Build history of the part. All positions in model axes, mm. Round coordinates to 2 decimals unless told otherwise and drop trailing zeros. Loops run counter-clockwise (first coordinate to the right, second up) from the corner with the lowest first, then second, coordinate; pieces in that order, holes last. Notation, with made-up numbers: (69, 54) - (110, 54) arc R22 cw to (110, 90) - close; hole circle Ø3 at (53, 68). An arc over 180 degrees is marked (long way). Put each result on its own line as item: value. Start each with the question number.
from build123d import *

# Parameters (mm, degrees)
F0_W     = 15
F0_H     = 5.08
F1_DEPTH = 5.08
F2_DEPTH = 25
F4_DEPTH = 50
F5_W     = 15
F5_H     = 5.08
F6_DEPTH = 5.08


# Not quite as in the source:
# - a feature names something its author has since deleted; it is built from what else it names


with BuildPart() as f1:
    # F0 (on Front) → F1 (new body)
    with BuildSketch(Plane.XZ):
        Polygon((-75.7, 0), (0, 0), (0, 50), (-104.7, 50), (-133.1023774395, 50), (-184.7, 50), (-184.7, 101.5976225605), (-184.7, 130), (-234.7, 130), (-234.7, 0), (-219.7, 0), (-210.7, 0), (-195.7, 0), (-186.7, 0), (-171.7, 0), (-162.7, 0), (-147.7, 0), (-138.7, 0), (-123.7, 0), (-114.7, 0), (-99.7, 0), (-90.7, 0), align=None)
        with Locations((-83.2, -2.54)):
            Rectangle(F0_W, F0_H)
        Polygon((-133.1023774395, 50), (-104.7, 50), (-184.7, 130), (-184.7, 101.5976225605), align=None)
        with Locations((-107.2, -2.54)):
            Rectangle(F0_W, F0_H)
        with Locations((-131.2, -2.54)):
            Rectangle(F0_W, F0_H)
        with Locations((-227.2, -2.54)):
            Rectangle(F0_W, F0_H)
        with Locations((-155.2, -2.54)):
            Rectangle(F0_W, F0_H)
        with Locations((-203.2, -2.54)):
            Rectangle(F0_W, F0_H)
        with Locations((-179.2, -2.54)):
            Rectangle(F0_W, F0_H)
    extrude(amount=F1_DEPTH)

    # F2 (add): a face of the model
    f2_faces = [f1.faces().sort_by_distance(p)[0] for p in [
        (-209.7, -2.54, 130),
    ]]
    extrude(f2_faces, amount=F2_DEPTH)

    # F3 (on face) → F4 (cut)
    with BuildSketch(Plane(origin=(0, 0, 0), x_dir=(1, 0, 0), z_dir=(0, 0, -1))):
        Polygon((0, 0), (0, 5.08), (-2.9329393675, 0), align=None)
    extrude(amount=-F4_DEPTH, mode=Mode.SUBTRACT)

    # F5 (on face) → F6 (join)
    with BuildSketch(Plane.XY.offset(50)):
        with Locations((-82.2, -2.54)):
            Rectangle(F5_W, F5_H)
    extrude(amount=F6_DEPTH)


solid = f1.part
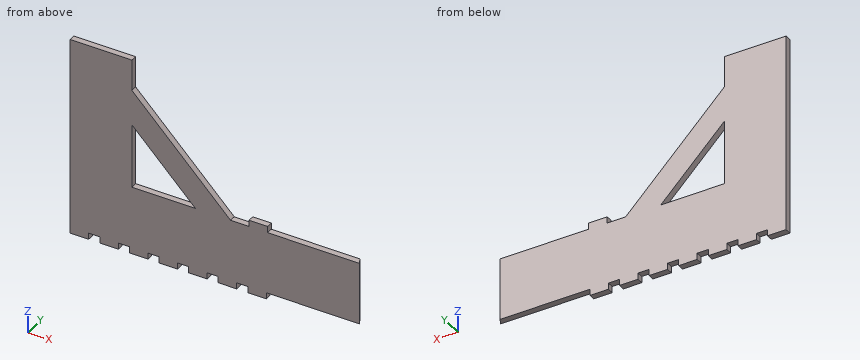
Item 1: Slice it at B-B (x = -150). Give the cut face in (y, z).
Item 2: Drill centre lines: probe 1 along Z at (x, y) = (-69.5, -2.9); probe 2 along X at (y, z) = (-1.5, 73.5); probe 3 along Z at (x, y) = (-149.5, -1.95). Where is each one in solid material? Low to high. Write a range as [from, to].
Item 3: Slice it at D-D (x = -43.5). Give the cut face in (y, z).
Item 4: Drop flat-ended pins along their axis: pin 1 Ø1 at (x, y) = (-36, -3) entering from -Z; pin 2 Ø1.5 at (x, y) = (-94, -3) entering from +Z; pin 3 Ø1.5 at (x, y) = (-84.5, -1.5) entering from +Z. Give the stop position or say it passes through.
Item 5: Slice it at C-C (z = 116). Give the cut face in (x, y).
Item 6: Slice it at A-A (z = 96). Give the cut face in (x, y), plus the area to 3 significant figures.
Computed values:
1. outline: (-5.08, -5.08) - (0, -5.08) - (0, 50) - (-5.08, 50) - close; (-5.08, 66.9) - (0, 66.9) - (0, 95.3) - (-5.08, 95.3) - close
2. probe 1: z = [0, 50]
2. probe 2: x = [-234.7, -184.7], [-156.6, -128.2]
2. probe 3: z = [-5.08, 50], [66.4, 94.8]
3. outline: (-5.08, 0) - (0, 0) - (0, 50) - (-5.08, 50) - close
4. pin 1: stops at z = 0
4. pin 2: stops at z = 50
4. pin 3: stops at z = 55.08
5. outline: (-234.7, -5.08) - (-170.7, -5.08) - (-170.7, 0) - (-234.7, 0) - close
6. outline: (-234.7, -5.08) - (-184.7, -5.08) - (-184.7, 0) - (-234.7, 0) - close; (-179.1, -5.08) - (-150.7, -5.08) - (-150.7, 0) - (-179.1, 0) - close
6. area: 398 mm^2
